The figure shows three views and two pictorial views of one solid part (mm, origin at its lowest corner). Answer the questions. A direction names the side the tool comes from. Coordinates: 2 decimals unless noted, no trailing zeros. Loops run counter-clockwise (first coordinate to the right, second up) from the corner with the lowest first, then second, coordinate; pieces in that order, holes last.
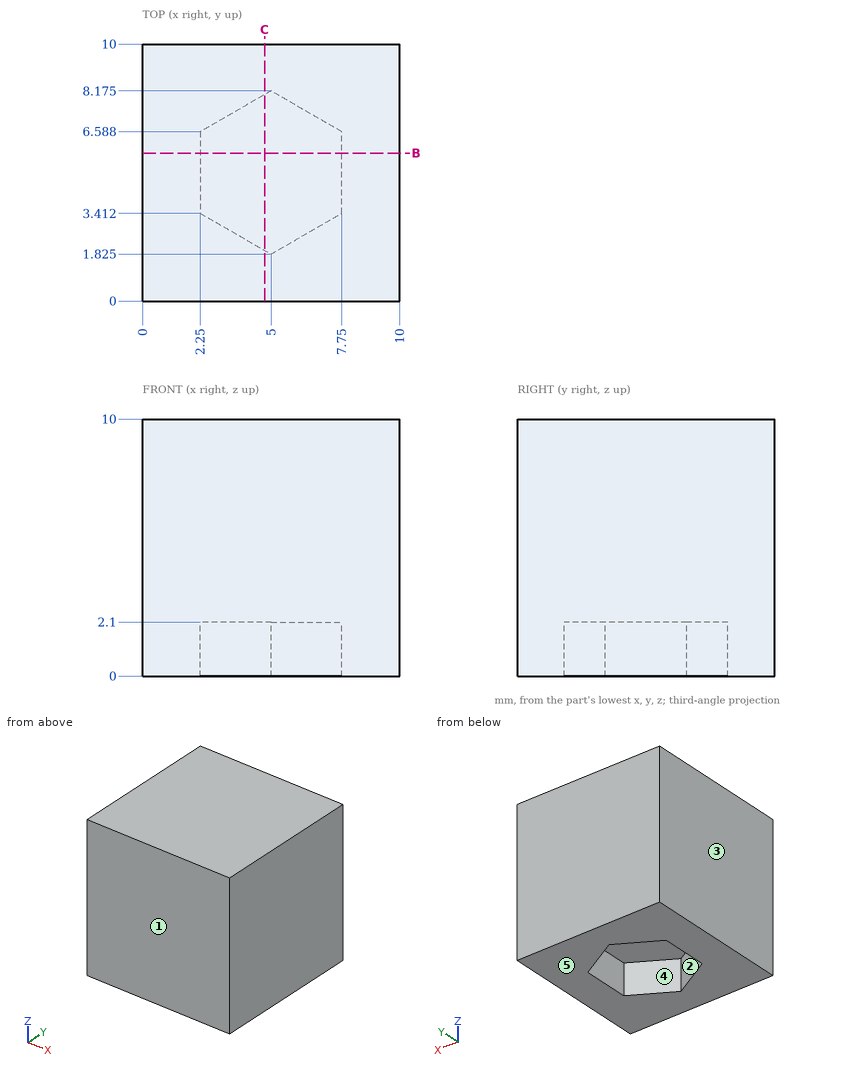
Q1. A cutting plane is placed at C-C (x = 4.75). Give the vertices of the cut face in (y, z).
Findings below:
outline: (0, 0) - (1.97, 0) - (1.97, 2.1) - (8.03, 2.1) - (8.03, 0) - (10, 0) - (10, 10) - (0, 10) - close
Q2. Determine the mould class of the marked faces 1, 2 and 3 for opening direction X: +X half, -X half, draft (parallel to the pull), parting line (faces both ways), or undercut.
Findings below:
face 1: draft
face 2: undercut
face 3: -X half
Q3. Which of the six approach directions +Z, -Z, +X, -X, +Y, -Y give full straight-line access (tool end or side, diameter ignored) to the marked faces 4 and 5?
Findings below:
face 4: -Z
face 5: -Z, +X, -X, +Y, -Y
Q4. Straight lines are drawn through the part: probe 1 along Z at (x, y) = (3, 4.75); probe 2 along X at (y, z) = (7, 1.75) (1 decimal). For each, find the intervals that lie inside material, in ascending order.
Findings below:
probe 1: z = 2.1 to 10
probe 2: x = 0 to 3, 7 to 10
Q5. A cutting plane is placed at B-B (y = 5.75). Give the vertices of the cut face in (x, z).
Findings below:
outline: (0, 0) - (2.25, 0) - (2.25, 2.1) - (7.75, 2.1) - (7.75, 0) - (10, 0) - (10, 10) - (0, 10) - close
